from build123d import *

# Parameters (mm, degrees)
SKETCH2_W                  = 132
SKETCH2_H                  = 232
PLATE_SIZE_DEPTH           = 4.4
SKETCH4_OUTSIDE_W          = 187.392
SKETCH4_OUTSIDE_H          = 287.392
OUTER_PROFILE_DEPTH        = 5.4
M3_CLEARANCE_HOLE1_D       = 3.5
F_18_0_18_DIAMETER_HOLE4_D = 18
M3_CLEARANCE_HOLE2_D       = 3.5
SKETCH13_W                 = 12.5
SKETCH13_H                 = 24
SERVO_CLEARANCE_DEPTH      = 5.4
M3_HEAD_CLEARANCE_HOLE3_D  = 4.7
M3_CLEARANCE_HOLE4_D       = 4
M3_CLEARANCE_HOLE5_D       = 3.7
SKETCH20_R                 = 9.017
CUT_EXTRUDE1_DEPTH         = 6.35


with BuildPart() as part:
    # Sketch2 → Plate Size (new body)
    with BuildSketch(Plane(origin=(0, 0, 0), x_dir=(1, 0, 0), z_dir=(0, 1, 0))):
        Rectangle(SKETCH2_W, SKETCH2_H)
    extrude(amount=PLATE_SIZE_DEPTH)

    # Sketch4 outside → Outer Profile (cut, through all)
    with BuildSketch(Plane(origin=(0, 0, 0), x_dir=(1, 0, 0), z_dir=(0, 1, 0))):
        Rectangle(SKETCH4_OUTSIDE_W, SKETCH4_OUTSIDE_H)
        with BuildLine():
            Line((-64.599996007, 76), (-47, 76))
            Line((-47, 76), (-47, 4))
            Line((-47, 4), (-62, 4))
            ThreePointArc((-62, 4), (-66, 0), (-62, -4))
            Line((-62, -4), (-47, -4))
            Line((-47, -4), (-47, -76))
            Line((-47, -76), (-64.599996007, -76))
            ThreePointArc((-64.599996007, -76), (-65.462483305, -76.493921289), (-65.472968926, -77.487768677))
            ThreePointArc((-65.472968926, -77.487768677), (0, -115.905117871), (65.472968926, -77.487768677))
            ThreePointArc((65.472968926, -77.487768677), (65.462483305, -76.493921289), (64.599996007, -76))
            Line((64.599996007, -76), (47, -76))
            Line((47, -76), (47, -4))
            Line((47, -4), (62, -4))
            ThreePointArc((62, -4), (66, 0), (62, 4))
            Line((62, 4), (47, 4))
            Line((47, 4), (47, 76))
            Line((47, 76), (64.599996007, 76))
            ThreePointArc((64.599996007, 76), (65.462483305, 76.493921289), (65.472968926, 77.487768677))
            ThreePointArc((65.472968926, 77.487768677), (0, 115.905117871), (-65.472968926, 77.487768677))
            ThreePointArc((-65.472968926, 77.487768677), (-65.462483305, 76.493921289), (-64.599996007, 76))
        make_face(mode=Mode.SUBTRACT)
    extrude(amount=OUTER_PROFILE_DEPTH, mode=Mode.SUBTRACT)

    # M3 Clearance Hole1 (through all)
    with Locations(Plane.XZ):
        with Locations((-55.999996141, 80.000001937), (55.999996141, 80.000001937), (-52.5, -85), (52.5, -85), (-55.999996141, 0), (55.999996141, 0)):
            Hole(M3_CLEARANCE_HOLE1_D / 2)

    # Ø18.0 (18) Diameter Hole4 (through all)
    with Locations(Plane.XZ):
        with Locations((0, -56), (0, 56)):
            Hole(F_18_0_18_DIAMETER_HOLE4_D / 2)

    # M3 Clearance Hole2 (through all)
    with Locations(Plane.XZ):
        with Locations((24.5, 87), (-15.5, 63), (-15.5, 87), (24.5, 63)):
            Hole(M3_CLEARANCE_HOLE2_D / 2)

    # Sketch13 → Servo Clearance (cut, through all)
    with BuildSketch(Plane(origin=(0, 0, 0), x_dir=(1, 0, 0), z_dir=(0, 1, 0))):
        with Locations((0, 88.75)):
            Rectangle(SKETCH13_W, SKETCH13_H)
    extrude(amount=SERVO_CLEARANCE_DEPTH, mode=Mode.SUBTRACT)

    # M3 Head Clearance Hole3 (through all)
    with Locations(Plane.XZ):
        with Locations((0, -103), (0, -74.5)):
            Hole(M3_HEAD_CLEARANCE_HOLE3_D / 2)

    # M3 Clearance Hole4 (through all)
    with Locations(Plane.XZ):
        with Locations((19.055000068, -73.5), (19.055000068, -88.75), (19.055000068, -104)):
            Hole(M3_CLEARANCE_HOLE4_D / 2)

    # M3 Clearance Hole5 (through all)
    with Locations(Plane.XZ):
        with Locations((37, -22.5), (-15.07, 10.08), (37, 5)):
            Hole(M3_CLEARANCE_HOLE5_D / 2)

    # Sketch20 → Cut-Extrude1 (cut)
    with BuildSketch(Plane(origin=(0, 4.4, 0), x_dir=(1, 0, 0), z_dir=(0, 1, 0))):
        Circle(SKETCH20_R)
    extrude(amount=-CUT_EXTRUDE1_DEPTH, mode=Mode.SUBTRACT)


solid = part.part
Design review of the part built by this model. Coordinates are the model's own, in mm. A direction names the side the tool comes from. Coordinates: 2 decimals unless noted, no trailing zeros. Loops run counter-clockwise (first coordinate to the right, second up) from the corner with the lowest first, then second, coordinate; pieces in that order, holes last. Notation, with made-up numbers: M 6,38.5 L 16,38.5 A33 cw 16,71.5 Z; hole C -36.75,23 d7. An arc over 180 degrees is marked long. Answer as CSV lines item,"result".
Item 1: For probe 1 along X at (y, z) = (2.7, -85); probe 2 along Z at (x, y) = (24, 1.8); probe 3 along Z at (x, y) = (52.5, 1.1), list the stretches that pass through material, from the lowest coordinate up.
Answer list:
probe 1,"-60.67 to -54.25, -50.75 to -6.25, 6.25 to 50.75, 54.25 to 60.67"
probe 2,"-111.96 to 61.32, 64.68 to 85.32, 88.68 to 111.96"
probe 3,"-94.47 to -86.75, -83.25 to -76, -4 to 4, 76 to 94.47"
Item 2: Add section C-C on x = -32. State the section outline as (y, z) points.
Answer list:
outline,"M 0,-108.74 L 4.4,-108.74 L 4.4,108.74 L 0,108.74 Z"
Item 3: For P1, Ø3, axis at x = 56, z = 80, coming from the -Y side; P2, Ø1, axis at y = 3.5, z = 49.5, coming from the +X side; P3, Ø2, axis at y = 1, z = -93.5, coming from the -X side; P4, Ø2, axis at x = 2.5, y = 3, coming from the -Z side, all flat-tipped, find the tip position at first contact; note any pin that passes through.
Answer list:
P1,"through"
P2,"x = 47"
P3,"x = -54.43"
P4,"z = -115.89"
Item 4: Machinability: for faces 1 (the face through (-6.25, 2, -89)), 2 (the face through (47, 2, -39)), 3 (the face through (-55, 2, 4)), which of the approach directions +Z, -Z, +X, -X, +Y, -Y give a long, thin tool a straight path to every point of the face, cutting with its end or side? Answer none if there is none.
Answer list:
face 1,"+Y, -Y"
face 2,"+X, +Y, -Y"
face 3,"-X, +Y, -Y"
Item 5: Add section B-B on y = 2.1. Count the separate pieces of the cut face and the enclosed holes in it, plus the area to 3 significant figures.
Answer list:
separate pieces,"1"
enclosed holes,"20"
area,"20,900 mm²"
Item 6: Add section A-A on z = -61. State the section outline as (x, y) points.
Answer list:
outline,"M -47,0 L -7.48,0 L -7.48,4.4 L -47,4.4 Z; M 7.48,0 L 47,0 L 47,4.4 L 7.48,4.4 Z"
Item 7: Add section D-D on z = 94. State the section outline as (x, y) points.
Answer list:
outline,"M -52.97,0 L 52.97,0 L 52.97,4.4 L -52.97,4.4 Z"
Item 8: The part is to be moulded in two halves that separate along Z. For faces 4 (the face through (14, 0, -2)), 5 (the face through (1.114, 2.169, -115.897)), 6 (the face through (55, 2, -4)), say which applies: pulls with the +Z half, pulls with the -Z half, needs draft (parallel to the pull), parting line crosses it, or undercut.
Answer list:
face 4,"needs draft"
face 5,"pulls with the -Z half"
face 6,"undercut"
